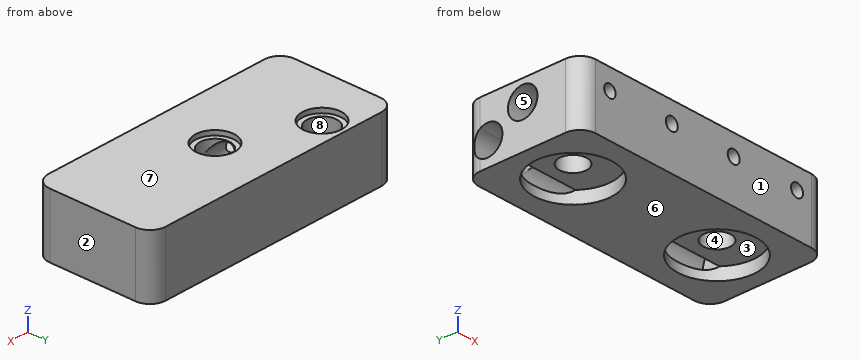
```python
from build123d import *

# Parameters (mm, degrees)
F0_W      = 170
F0_H      = 75
F1_DEPTH  = 40
F2_R      = 10
F3_R      = 25
F3_R_2    = 8.75
F6_DEPTH  = 8
F7_DEPTH  = 27
F4_R      = 9.5
F8_DEPTH  = 160
F5_R      = 12.5
F5_R_2    = 9.5
F9_DEPTH  = 3
F10_DEPTH = 13
F11_DEPTH = 25
F12_R     = 4
F12_R_2   = 4.15
F13_DEPTH = 35


with BuildPart() as f1:
    # F0 (on Top) → F1 (new body)
    with BuildSketch(Plane.XY):
        with Locations((-85, 37.5)):
            Rectangle(F0_W, F0_H)
    extrude(amount=F1_DEPTH)

    # F2
    f2_edges = [f1.edges().sort_by_distance(p)[0] for p in [
        (0, 0, 20),
        (0, 75, 20),
        (-170, 0, 20),
        (-170, 75, 20),
    ]]
    fillet(f2_edges, radius=F2_R)

    # F3 (on face) → F6 (cut)
    with BuildSketch(Plane(origin=(0, 0, 0), x_dir=(1, 0, 0), z_dir=(0, 0, -1))):
        with Locations((-135, -37.5)):
            Circle(F3_R)
        with Locations((-135, -37.5)):
            Circle(F3_R_2, mode=Mode.SUBTRACT)
        with Locations((-35, -37.5)):
            Circle(F3_R)
        with Locations((-35, -37.5)):
            Circle(F3_R_2, mode=Mode.SUBTRACT)
    extrude(amount=-F6_DEPTH, mode=Mode.SUBTRACT)

    # F7 (cut): faces of the model
    f7_faces = [f1.faces().sort_by_distance(p)[0] for p in [
        (-135, 37.5, 0),
        (-35, 37.5, 0),
    ]]
    extrude(f7_faces, amount=-F7_DEPTH, mode=Mode.SUBTRACT)

    # F4 (on face) → F8 (cut)
    with BuildSketch(Plane(origin=(-170, 0, 0), x_dir=(0, -1, 0), z_dir=(-1, 0, 0))):
        with Locations((-37.5, 27)):
            Circle(F4_R)
        with BuildLine():
            ThreePointArc((-65, 6.9222527893), (-55.3766894978, 6.7009036637), (-50.5, 15))
            ThreePointArc((-50.5, 15), (-55.3766894978, 23.2990963363), (-65, 23.0777472107))
            Line((-65, 23.0777472107), (-65, 6.9222527893))
        make_face()
        with BuildLine():
            Line((-65, 6.9222527893), (-65, 23.0777472107))
            ThreePointArc((-65, 23.0777472107), (-69.5, 15), (-65, 6.9222527893))
        make_face()
    extrude(amount=-F8_DEPTH, mode=Mode.SUBTRACT)

    # F5 (on face) → F9 (cut)
    with BuildSketch(Plane.XY.offset(40)):
        with Locations((-135, 60)):
            Circle(F5_R)
        with Locations((-135, 60)):
            Circle(F5_R_2, mode=Mode.SUBTRACT)
        with Locations((-85, 37.5)):
            Circle(F5_R)
        with Locations((-85, 37.5)):
            Circle(F5_R_2, mode=Mode.SUBTRACT)
    extrude(amount=-F9_DEPTH, mode=Mode.SUBTRACT)

    # F10 (cut): a face of the model
    f10_faces = [f1.faces().sort_by_distance(p)[0] for p in [
        (-85, 37.5, 40),
    ]]
    extrude(f10_faces, amount=-F10_DEPTH, mode=Mode.SUBTRACT)

    # F11 (cut): a face of the model
    f11_faces = [f1.faces().sort_by_distance(p)[0] for p in [
        (-135, 60, 40),
    ]]
    extrude(f11_faces, amount=-F11_DEPTH, mode=Mode.SUBTRACT)

    # F12 (on face) → F13 (cut)
    with BuildSketch(Plane.XZ):
        with Locations((-150, 27)):
            Circle(F12_R)
        with Locations((-107, 27)):
            Circle(F12_R_2)
        with Locations((-64, 27)):
            Circle(F12_R_2)
        with Locations((-20, 27)):
            Circle(F12_R_2)
    extrude(amount=-F13_DEPTH, mode=Mode.SUBTRACT)


solid = f1.part
```
The listing builds one solid part. Answer for the finished solid, in the listing's coordinates (mm). Face numbers are marked on the shaded views. A direction names the side the tool comes from. Coordinates: 2 decimals unless noted, no trailing zeros. Loops run counter-clockwise (first coordinate to the right, second up) from the corner with the lowest first, then second, coordinate; pieces in that order, holes last. Notation, with made-up numbers: M 18.25,70 L 26.25,70 A15 cw 26.25,77 Z; hole C -16.5,38 d2. An arc over 180 degrees is marked long. Answer as a JSON object with one key per item and string values. Group by question number.
Item 1: Section A-A (y = 37.5) is taken. Give the number of separate pieces and of enclosed holes in the cut face, and give its area (3 significant figures).
Item 2: Which of the six approach directions +Z, -Z, +X, -X, +Y, -Y give full straight-line access (tool end or side, diameter ignored) to the marked faces 4, 5, 6, 7 and 8?
Item 3: Section D-D (x = -56) is taken. Write down the section's boundary in (y, z), and give its area (3 significant figures).
Item 4: Determine the mould class of the marked faces 1, 2 and 3 for opening direction Y: +Y half, -Y half, draft (parallel to the pull), parting line (faces both ways), or undercut.
Item 5: Section B-B (x = -85) is taken. Write down the section's boundary in (y, z), and give its area (3 significant figures).
Item 6: Consider L1, parallel to X at y = 16, z = 27; L2, parallel to X at y = 37.5, z = 4; L3, parallel to Y at x = -35, z = 5.5. Determine where each line is inside the solid, lowest interval first.
Item 7: Each of these flat-tipped pins is pushed along its axis until it touches: P1, Ø7.5, axis at x = -20, z = 27, coming from the -Y side; P2, Ø9.5, axis at x = -64, z = 27, coming from the -Y side; P3, Ø15, axis at x = -85, y = 37.5, coming from the +Z side. Where does it stop, or does it pass through?
Solved:
{
 "1": {"separate pieces": "4", "enclosed holes": "0", "area": "2,540 mm2"},
 "2": {"face 4": "-Z", "face 5": "-X", "face 6": "-Z, +X, -X, +Y, -Y", "face 7": "+Z, +X, -X, +Y, -Y", "face 8": "+Z"},
 "3": {"outline": "M 0,0 L 23.94,0 L 23.94,8 L 51.06,8 L 51.06,0 L 75,0 L 75,40 L 0,40 Z; hole C 37.5,27 d19; hole C 60,15 d19", "area": "2,220 mm2"},
 "4": {"face 1": "-Y half", "face 2": "draft", "face 3": "undercut"},
 "5": {"outline": "M 0,0 L 75,0 L 75,40 L 50,40 L 50,37 L 47,37 L 47,27 A9.5 cw 28,27 L 28,37 L 25,37 L 25,40 L 0,40 Z; hole C 60,15 d19", "area": "2,310 mm2"},
 "6": {"L1": "x = -170 to -154, -146 to -111.15, -102.85 to -68.15, -59.85 to -24.15, -15.85 to 0", "L2": "x = -170 to -160, -110 to -60, -10 to 0", "L3": "y = 0 to 12.5, 62.5 to 75"},
 "7": {"P1": "stops at y = 46.23", "P2": "stops at y = 0", "P3": "stops at z = 21.17"}
}
